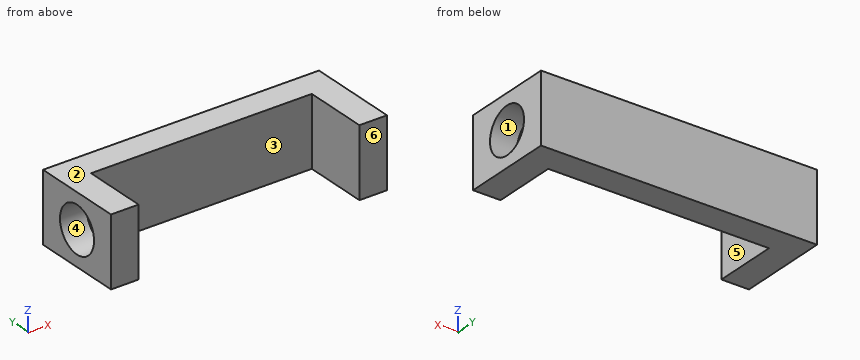
```python
from build123d import *

# Parameters (mm, degrees)
SKETCH1_W               = 30
SKETCH1_H               = 10
BOSS_EXTRUDE1_DEPTH     = 3.75
CUT_EXTRUDE1_REACH      = 9.5
SKETCH2_W               = 24
SKETCH2_H               = 7
SKETCH4_R               = 2.5
CUT_EXTRUDE2_DEPTH      = 16
CUT_EXTRUDE2_DEPTH_BACK = 16
BOSS_EXTRUDE2_START     = -3
SKETCH5_R               = 2.5
BOSS_EXTRUDE2_DEPTH     = 0.1
BOSS_EXTRUDE3_START     = -3
SKETCH6_R               = 2.5
BOSS_EXTRUDE3_DEPTH     = 0.1
SKETCH7_W               = 24
SKETCH7_H               = 3
BOSS_EXTRUDE4_DEPTH     = 7.5


with BuildPart() as part:
    # Sketch1 → Boss-Extrude1 (new body, symmetric)
    with BuildSketch(Plane.XY):
        Rectangle(SKETCH1_W, SKETCH1_H)
    extrude(amount=BOSS_EXTRUDE1_DEPTH, both=True)

    # Sketch2 → Cut-Extrude1 (cut, up to next)
    with BuildSketch(Plane.XY.offset(3.75), mode=Mode.PRIVATE) as cut_extrude1_sk1:
        with Locations((0, -1.5)):
            Rectangle(SKETCH2_W, SKETCH2_H)
    cut_extrude1_tool1 = extrude(cut_extrude1_sk1.sketch, amount=-CUT_EXTRUDE1_REACH, mode=Mode.PRIVATE) & part.part
    add(cut_extrude1_tool1.solids().sort_by_distance((0, -1.5, 3.75))[0], mode=Mode.SUBTRACT)

    # Sketch4 → Cut-Extrude2 (cut, two sides)
    with BuildSketch(Plane(origin=(0, 0, 0), x_dir=(0, 0, -1), z_dir=(1, 0, 0))) as cut_extrude2_sk:
        Circle(SKETCH4_R)
    extrude(amount=CUT_EXTRUDE2_DEPTH, mode=Mode.SUBTRACT)
    extrude(cut_extrude2_sk.sketch, amount=-CUT_EXTRUDE2_DEPTH_BACK, mode=Mode.SUBTRACT)

    # Sketch5 → Boss-Extrude2 (add)
    with BuildSketch(Plane(origin=(15, 0, 0), x_dir=(0, 0, -1), z_dir=(1, 0, 0)).offset(BOSS_EXTRUDE2_START)):
        Circle(SKETCH5_R)
    extrude(amount=BOSS_EXTRUDE2_DEPTH)

    # Sketch6 → Boss-Extrude3 (add)
    with BuildSketch(Plane.ZY.offset(15).offset(BOSS_EXTRUDE3_START)):
        Circle(SKETCH6_R)
    extrude(amount=BOSS_EXTRUDE3_DEPTH)

    # Sketch7 → Boss-Extrude4 (add)
    with BuildSketch(Plane(origin=(0, 0, -3.75), x_dir=(-1, 0, 0), z_dir=(0, 0, -1))):
        with Locations((0, 3.5)):
            Rectangle(SKETCH7_W, SKETCH7_H)
    extrude(amount=-BOSS_EXTRUDE4_DEPTH)


solid = part.part
```
Geometry check sheet. Reference: the model listing, model coordinates, mm. Face numbers are marked on the shaded views. A direction names the side the tool comes from. Give positions to 0.01 mm unless a question says otherwise; leave off trailing zeros. Loops run counter-clockwise (first coordinate to the right, second up) from the corner with the lowest first, then second, coordinate; pieces in that order, holes last. Notation, with made-up numbers: (-38.75, -4.5) - (-12.75, -4.5) arc R35 cw to (-12.75, 32.5) - close; hole circle Ø10 at (80.5, 35.25). An arc over 180 degrees is marked (long way). Use CSV: the item, a comma, the result in double quotes. Start each with the question number.
Q1. Section check C-C, the plane z = 0. Record the cut outline in (x, y).
Q2. Scan lines: probe 1 along Y at (x, z) = (14.25, 0); probe 2 along X at (y, z) = (0, -3.5); probe 3 along Y at (x, z) = (-1.25, 3). Record each from-to range of solid material in increasing order. Write a range as from..to.
Q3. Access from +Z, -Z, +X, -X, +Y, -Y to the whole of each face (thin tool, end or side, straight path). Record for the marked faces 5 and 6.
Q4. Section check A-A, the plane y = 0. Record the cut outline in (x, z).
Q5. Section check B-B, the plane z = -2. Record the cut outline in (x, y).
Q6. Release check for a two-part mould opening along Z. For the marked faces 1, 2, 3 and 4 record: +Z half, -Z half, draft (parallel to the pull), parting line (faces both ways), or undercut.
Q7. Section check D-D, the plane x = -3.5. Record the cut outline in (y, z), and give its area (3 significant figures).
Q8. Go/stop test with flat-tipped pins: pin 1 Ø4 at (x, z) = (-4.5, -1.5) entering from -Y; pin 2 Ø4.5 at (y, z) = (0, 0) entering from -X; pin 3 Ø2.5 at (y, z) = (1, 1) entering from -X; pin 4 Ø1.5 at (y, z) = (-1, -0.5) entering from +X. Record where each tip stops, or that it passes through.
Findings below:
1,outline,"(-15, -5) - (-12, -5) - (-12, 2) - (12, 2) - (12, -5) - (15, -5) - (15, -2.5) - (12.1, -2.5) - (12.1, 2.5) - (15, 2.5) - (15, 5) - (-15, 5) - (-15, 2.5) - (-12.1, 2.5) - (-12.1, -2.5) - (-15, -2.5) - close"
2,probe 1,"y = -5..-2.5, 2.5..5"
2,probe 2,"x = -15..-12, 12..15"
2,probe 3,"y = 2..5"
3,face 5,"+Z, -Z, -Y"
3,face 6,"+Z, -Z, +X, -X, -Y"
4,outline,"(-15, -3.75) - (-12, -3.75) - (-12, 3.75) - (-15, 3.75) - (-15, 2.5) - (-12.1, 2.5) - (-12.1, -2.5) - (-15, -2.5) - close; (12, -3.75) - (15, -3.75) - (15, -2.5) - (12.1, -2.5) - (12.1, 2.5) - (15, 2.5) - (15, 3.75) - (12, 3.75) - close"
5,outline,"(-15, -5) - (-12, -5) - (-12, 2) - (12, 2) - (12, -5) - (15, -5) - (15, -1.5) - (12.1, -1.5) - (12.1, 1.5) - (15, 1.5) - (15, 5) - (-15, 5) - (-15, 1.5) - (-12.1, 1.5) - (-12.1, -1.5) - (-15, -1.5) - close"
6,face 1,"undercut"
6,face 2,"+Z half"
6,face 3,"draft"
6,face 4,"undercut"
7,outline,"(2, -3.75) - (5, -3.75) - (5, 3.75) - (2, 3.75) - close"
7,area,"22.5 mm^2"
8,pin 1,"stops at y = 2"
8,pin 2,"stops at x = -12.1"
8,pin 3,"stops at x = -15"
8,pin 4,"stops at x = 12.1"
